For this review, take the finished solid that the model builds, in its own axes (mm). Face numbers are marked on the shaded views. A direction names the side the tool comes from. Give positions to 0.01 mm unless a question says otherwise; leave off trailing zeros. Order: outer loops, then holes, each group sorted by start corner. A loop starts at its lowest first (then second) coordinate and runs counter-clockwise, first axis right, second up. Notation, with made-up numbers: M 22,-25 L 28,-25 A18 cw 28,6 Z; hole C 54,49 d2. An arc over 180 degrees is marked long. Answer as CSV lines item,"result". Start each with the question number.
1. Machinability: for the marked faces 1, 2 and 3, which of the approach directions +Z, -Z, +X, -X, +Y, -Y give a long, thin tool a straight path to every point of the face, cutting with its end or side? Answer none if there is none.
2. Mouldability with a two-part tool opening along Z and no side actions: class the marked faces 4, 5 and 6 as pulls with the +Z half, pulls with the -Z half, needs draft (parallel to the pull), parting line crosses it, or undercut.
3. We need section D-D, the plane x = 15.5. Give the boundary of the cut face in (y, z), and give its area (3 significant figures).
4. We need section C-C, the plane y = 3.75. Give the boundary of the cut face in (x, z), and give its area (3 significant figures).
5. For line 1 along Z through (x, y) = (15.5, -6.05); line 2 along Z through (x, y) = (15.5, -2); line 3 along Z through (x, y) = (15, 3.75), list the stretches that pass through material, from the lowest coordinate up.
6. We need section A-A, the plane x = 0. Give the boundary of the cut face in (y, z).
7. We need section B-B, the plane z = -15.5. Give the boundary of the cut face in (x, y), and give its area (3 significant figures).
8. Clearance check with a flat-ended pin moving along its axis: P1, Ø1.5, axis at x = -15, z = -13, coming from the +Y side. State where the tip first meets the part, or that it passes through.
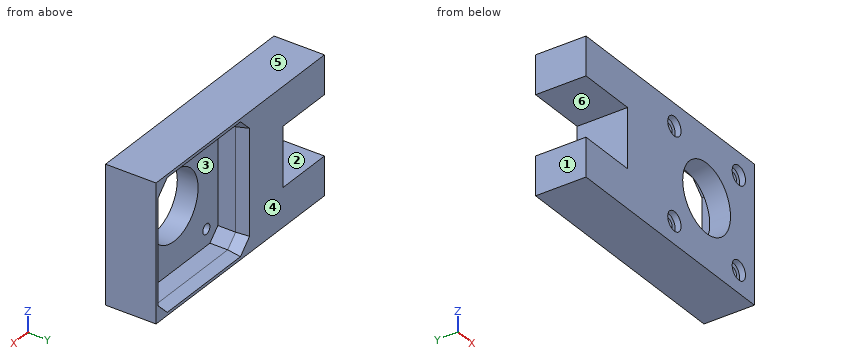
Autodesk Inventor part; units mm, degrees
ref_plane "YZ Plane" through (0, 0, 0) normal (1, 0, 0) x (0, 1, 0)
ref_plane "XZ Plane" through (0, 0, 0) normal (0, 1, 0) x (-1, 0, 0)
ref_plane "XY Plane" through (0, 0, 0) normal (0, 0, 1) x (1, 0, 0)
sketch "Sketch1" plane through (0, 0, 0) normal (0, 1, 0) x (-1, 0, 0)
  line L0 (-21, 21) -> (21, 21)
  line L1 (21, 21) -> (21, -21)
  line L2 (21, -21) -> (-21, -21)
  line L3 (-21, -21) -> (-21, 21)
  line L4 (-21, 21) -> (21, -21) construction
  line L5 (21, 21) -> (-21, -21) construction
  circle A0 centre (15.5, -15.5) radius 1.7
  circle A1 centre (-15.5, -15.5) radius 1.7
  line L6 (15.5, -15.5) -> (-15.5, -15.5) construction
  circle A2 centre (15.5, 15.5) radius 1.7
  line L7 (15.5, 15.5) -> (-15.5, 15.5) construction
  circle A3 centre (-15.5, 15.5) radius 1.7
  line L8 (-23, 23) -> (23, 23)
  line L9 (23, 23) -> (23, -23)
  line L10 (23, -23) -> (-23, -23)
  line L11 (-23, -23) -> (-23, 23)
  circle A4 centre (0, 0) radius 11.5
  line L12 (23, 23) -> (-23, 23)
  circle A5 centre (15.5, 15.5) radius 3.2
  circle A6 centre (-15.5, 15.5) radius 3.2
  circle A7 centre (-15.5, -15.5) radius 3.2
  circle A8 centre (15.5, -15.5) radius 3.2
  line L13 (23, 23) -> (58, 23)
  line L14 (58, 23) -> (58, 10)
  line L15 (58, 10) -> (23, 10)
  line L16 (23, 10) -> (23, 23)
  line L17 (23, -23) -> (58, -23)
  line L18 (58, -23) -> (58, -10)
  line L19 (58, -10) -> (23, -10)
  line L20 (23, -10) -> (23, -23)
  line L21 (38, -10) -> (38, 10)
  dimension "d20" = 31
  dimension "d21" = 42
  dimension "d22" = 42
  dimension "d23" = 3.4
  dimension "d24" = 3.4
  dimension "d25" = 3.4
  dimension "d26" = 31
  dimension "d27" = 3.4
  dimension "d28" = 2
  dimension "d29" = 2
  dimension "d30" = 2
  dimension "d31" = 2
  dimension "d32" = 23
  dimension "d60" = 1.5
  dimension "d61" = 1.5
  dimension "d62" = 1.5
  dimension "d63" = 1.5
  dimension "d74" = 15
  dimension "d75" = 20
  dimension "d76" = 20
extrude "Extrusion1" add sketch "Sketch1" along normal blind 10 contours L8 L9 L10 L11 | L13 L14 L15 L9 | L15 L21 L19 L9 | L9 L19 L18 L17
extrude "Extrusion2" add sketch "Sketch1" against normal blind 7 contours L0 L1 L2 L3 | L8 L9 L10 L11 | L13 L14 L15 L9 | L15 L21 L19 L9 | L9 L19 L18 L17 | A5 | A6 | A7 | A8
chamfer "Chamfer1" distance 3.8 angle 45 4 edges at (-21, 5, 21) (-21, 5, -21) (21, 5, -21) (21, 5, 21)
chamfer "Chamfer2" distance 1 distance2 4 8 edges at (0, 10, -21) (19.1, 10, -19.1) (21, 10, 0) (19.1, 10, 19.1) (0, 10, 21) (-21, 10, 0) (-19.1, 10, -19.1) (-19.1, 10, 19.1) measured on face at (-26.6667, 10, 3.3333)
extrude "Extrusion3" cut sketch "Sketch1" along normal blind 2 from surface at -7 contours A3 | A5 | A6 | A7 | A8
equation "\"d24\" = d23"
equation "\"d25\" = d23"
equation "\"d26\" = d20"
equation "\"d27\" = d23"
equation "\"d29\" = d28"
equation "\"d30\" = d31"
properties part number "Z Stepper Holder"
Result set:
1,face 1,"+Z, -Z, -X, +Y, -Y"
1,face 2,"-X, +Y, -Y"
1,face 3,"+Y"
2,face 4,"needs draft"
2,face 5,"pulls with the +Z half"
2,face 6,"undercut"
3,outline,"M -7,-23 L 10,-23 L 10,-22 L 6,-21 L 0,-21 L 0,-17.2 L -5,-17.2 L -5,-18.7 L -7,-18.7 Z; M -7,-12.3 L -5,-12.3 L -5,-13.8 L 0,-13.8 L 0,13.8 L -5,13.8 L -5,12.3 L -7,12.3 Z; M -7,18.7 L -5,18.7 L -5,17.2 L 0,17.2 L 0,21 L 6,21 L 10,22 L 10,23 L -7,23 Z"
3,area,"298 mm2"
4,outline,"M -58,-23 L 23,-23 L 23,23 L -58,23 L -58,10 L -38,10 L -38,-10 L -58,-10 Z; hole M -21,-17.2 L -17.2,-21 L 17.2,-21 L 21,-17.2 L 21,17.2 L 17.2,21 L -17.2,21 L -21,17.2 Z"
4,area,"1,590 mm2"
5,line 1,"-23 to -18.7, -12.3 to 12.3, 18.7 to 23"
5,line 2,"-23 to -17.2, -13.8 to 13.8, 17.2 to 23"
5,line 3,"-23 to -21, 21 to 23"
6,outline,"M -7,-23 L 10,-23 L 10,-22 L 6,-21 L 0,-21 L 0,-11.5 L -7,-11.5 Z; M -7,11.5 L 0,11.5 L 0,21 L 6,21 L 10,22 L 10,23 L -7,23 Z"
7,outline,"M -58,-7 L -18.7,-7 L -18.7,-5 L -17.2,-5 L -17.2,0 L -21,0 L -21,6 L -22,10 L -58,10 Z; M -13.8,-5 L -12.3,-5 L -12.3,-7 L 12.3,-7 L 12.3,-5 L 13.8,-5 L 13.8,0 L -13.8,0 Z; M 17.2,-5 L 18.7,-5 L 18.7,-7 L 23,-7 L 23,10 L 22,10 L 21,6 L 21,0 L 17.2,0 Z"
7,area,"893 mm2"
8,P1,"y = 0"
